```python
from build123d import *

# Parameters (mm, degrees)
HEX_BLANK_DEPTH                  = 2.4
NOMINAL_THREAD_ENVELOPE_START    = -1
SKETCH_NOMINAL_THREAD_ENVELOPE_R = 1.52
NOMINAL_THREAD_ENVELOPE_DEPTH    = 4.4


with BuildPart() as part:
    # Sketch_Hex_blank → Hex_blank (new body)
    with BuildSketch(Plane.XY):
        Polygon((3.175426481, 0), (1.58771324, 2.75), (-1.58771324, 2.75), (-3.175426481, 0), (-1.58771324, -2.75), (1.58771324, -2.75), align=None)
    extrude(amount=HEX_BLANK_DEPTH)

    # Sketch_Nominal_thread_envelope → Nominal_thread_envelope (cut)
    with BuildSketch(Plane.XY.offset(NOMINAL_THREAD_ENVELOPE_START)):
        Circle(SKETCH_NOMINAL_THREAD_ENVELOPE_R)
    extrude(amount=NOMINAL_THREAD_ENVELOPE_DEPTH, mode=Mode.SUBTRACT)


solid = part.part
```
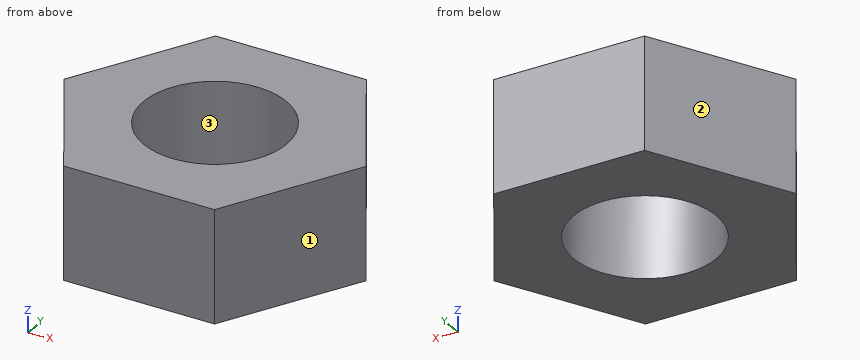
The model under review builds one solid part; all positions refer to its coordinate system, in mm. Face numbers are marked on the shaded views. Round coordinates to 2 decimals unless told otherwise and drop trailing zeros. Loops run counter-clockwise (first coordinate to the right, second up) from the corner with the lowest first, then second, coordinate; pieces in that order, holes last. Notation, with made-up numbers: (-25.75, 86) -> (-13.75, 86) arc R12 ccw to (-13.75, 101) -> close; hole circle Ø6 at (54.5, -9). An arc over 180 degrees is marked (long way). Answer as a JSON object with one key per item and string values. Group by question number.
1) We need section D-D on y = 2.25. Write out the cut boundary in (x, z).
2) For line 1 (Y direction, x = 0, z = 1.45); line 2 (X direction, y = 0.2, z = 2.25); line 3 (X direction, y = -1.3, z = 0.3), list the stretches that pass through material, from the lowest coordinate up. Write a range as [from, to].
3) We need section C-C on y = -0.7. Write out the cut boundary in (x, z), then the cut area to 3 significant figures.
4) We need section A-A on z = 2. Write out the cut boundary in (x, y), then the cut area to 3 significant figures.
5) We need section B-B on x = 0.75. Write out the cut boundary in (y, z).
6) Mouldability with a two-part tool opening along X and no side actions: class the marked faces 1, 2 and 3 as released by +X, released by -X, zero draft, split by the parting line, or undercut.
7) For pin 1 Ø1 at (x, y) = (-1, -1.5) entering from -Z, flat-tipped, find the tip position at first contact; note if it passes through.
Result set:
{
 "1": {"outline": "(-1.88, 0) -> (1.88, 0) -> (1.88, 2.4) -> (-1.88, 2.4) -> close"},
 "2": {"line 1": "[-2.75, -1.52], [1.52, 2.75]", "line 2": "[-3.06, -1.51], [1.51, 3.06]", "line 3": "[-2.42, -0.79], [0.79, 2.42]"},
 "3": {"outline": "(-2.77, 0) -> (-1.35, 0) -> (-1.35, 2.4) -> (-2.77, 2.4) -> close; (1.35, 0) -> (2.77, 0) -> (2.77, 2.4) -> (1.35, 2.4) -> close", "area": "6.83 mm²"},
 "4": {"outline": "(-3.18, 0) -> (-1.59, -2.75) -> (1.59, -2.75) -> (3.18, 0) -> (1.59, 2.75) -> (-1.59, 2.75) -> close; hole circle Ø3.04 at (0, 0)", "area": "18.9 mm²"},
 "5": {"outline": "(-2.75, 0) -> (-1.32, 0) -> (-1.32, 2.4) -> (-2.75, 2.4) -> close; (1.32, 0) -> (2.75, 0) -> (2.75, 2.4) -> (1.32, 2.4) -> close"},
 "6": {"face 1": "released by +X", "face 2": "released by -X", "face 3": "undercut"},
 "7": {"pin 1": "z = 0"}
}
